Check sheet for the modelled part. Datum: model origin and axes. Units: mm. Face numbers are marked on the shaded views. Give positions to 0.01 mm unless a question says otherwise; leave off trailing zeros. Loops run counter-clockwise (first coordinate to the right, second up) from the corner with the lowest first, then second, coordinate; pieces in that order, holes last. Notation, with made-up numbers: (69.25, -23.75) -> (105.25, -23.75) arc R23 cw to (105.25, 7.25) -> close; hole circle Ø7 at (13, 84.25). An arc over 180 degrees is marked (long way). Write each question's results on one line, items separated by ' | '. Start each with the question number.
1. Cross-section at A-A on x = 0. Record the boundary of the cut face in (y, z) (3 decimals), and give its area (3 significant figures).
2. Mould release check, pull along Z, two halves, no side actions. Record for the marked faces 1, 2 and 3: +Z half, -Z half, draft (parallel to the pull), parting line (faces both ways), or undercut.
3. Material ranges on L1, parallel to Y at x = -12.2, z = 0; L2, parallel to X at y = 143.5, z = 0; L3, parallel to Y at x = -11, z = -7, recorded low to high. Write a range as from..to.
4. Gauge pin test, flat ends, axial feed: pin 1 Ø5 at (x, y) = (1.5, 170.5) entering from -Z; pin 2 Ø12 at (x, y) = (-1, 62) entering from +Z; pin 3 Ø9 at (x, z) = (-1.5, 1.5) entering from +Y. Record the tip position at first contact, or that the pin passes through.
5. Cross-section at B-B on y = 146.5. Record the boundary of the cut face in (x, z).
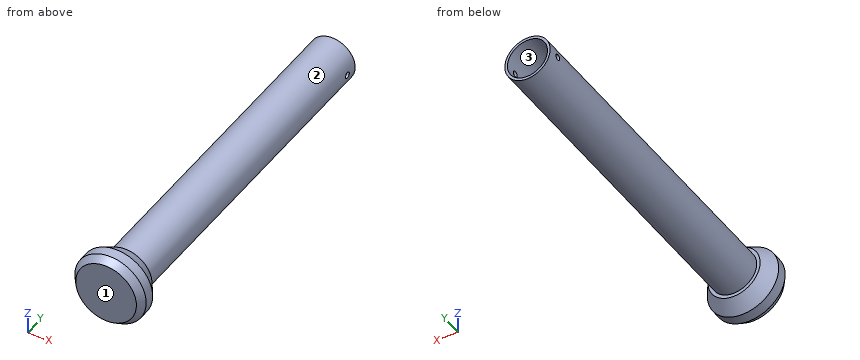
from build123d import *

# Parameters (mm, degrees)
SKETCH1_R               = 12.7
SKETCH1_R_2             = 11.227
BOSS_EXTRUDE1_DEPTH     = 205
CUT_EXTRUDE1_DEPTH      = 207.942020866
CUT_EXTRUDE1_DEPTH_BACK = 207.942020866
SKETCH3_R               = 1.7


with BuildPart() as part:
    # Sketch1 → Boss-Extrude1 (new body)
    with BuildSketch(Plane(origin=(0, 0, 0), x_dir=(1, 0, 0), z_dir=(0, 1, 0))):
        with Locations(Location((0, 0, 0), (0, 0, 90))):
            Circle(SKETCH1_R)
        with Locations(Location((0, 0, 0), (0, 0, 90))):
            Circle(SKETCH1_R_2, mode=Mode.SUBTRACT)
    extrude(amount=BOSS_EXTRUDE1_DEPTH)

    # Sketch2 → Revolve1 (revolve)
    with BuildSketch(Plane.XY, mode=Mode.PRIVATE) as revolve1_sk:
        Polygon((0, 0), (17, 0), (20, 4), (20, 9.9), (14.605, 18), (0, 18), align=None)
    revolve(revolve1_sk.sketch.rotate(Axis((0, -10, 0), (0, 1, 0)), 90), axis=Axis((0, -10, 0), (0, 1, 0)))

    # Sketch3 → Cut-Extrude1 (cut, two sides: drawn at the far end of the back side and taken through both)
    with BuildSketch(Plane(origin=(0, 0, 0), x_dir=(0, 0, -1), z_dir=(1, 0, 0)).offset(-CUT_EXTRUDE1_DEPTH_BACK)):
        with Locations((0, 198)):
            Circle(SKETCH3_R)
    extrude(amount=CUT_EXTRUDE1_DEPTH + CUT_EXTRUDE1_DEPTH_BACK, mode=Mode.SUBTRACT)


solid = part.part
Geometry says:
1) outline: (0, -17) -> (4, -20) -> (9.9, -20) -> (18, -14.605) -> (18, -12.7) -> (205, -12.7) -> (205, -11.227) -> (18, -11.227) -> (18, 11.227) -> (205, 11.227) -> (205, 12.7) -> (18, 12.7) -> (18, 14.605) -> (9.9, 20) -> (4, 20) -> (0, 17) -> close | area: 1,220 mm^2
2) face 1: draft | face 2: parting line | face 3: undercut
3) L1: 0..196.3, 199.7..205 | L2: -12.7..-11.23, 11.23..12.7 | L3: 0..18
4) pin 1: z = -12.7 | pin 2: z = 12.7 | pin 3: y = 18
5) outline: circle Ø25.4 at (0, 0); hole circle Ø22.45 at (0, 0)
